Autodesk Fusion 360 part; units mm, degrees
sketch "Sketch1" plane through (0, 0, 0) normal (0, 0, 1) x (1, 0, 0)
  line L0 (110, 0) -> (80, 0)
  line L1 (80, 0) -> (80, 20)
  line L2 (80, 20) -> (40, 20)
  line L3 (40, 20) -> (40, 0)
  line L4 (0, 0) -> (40, 0)
  line L5 (80, 0) -> (110, 0)
  line L6 (110, 0) -> (110, 10)
  line L7 (110, 10) -> (90, 10)
  line L8 (90, 10) -> (90, 50)
  line L9 (90, 50) -> (20, 50)
  line L10 (0, 0) -> (0, 10)
  line L11 (0, 10) -> (20, 10)
  line L12 (20, 10) -> (20, 50)
  dimension "d1" = 110
  dimension "d2" = 30
  dimension "d3" = 20
  dimension "d4" = 40
  dimension "d5" = 10
  dimension "d6" = 20
  dimension "d7" = 70
  dimension "d8" = 10
  dimension "d9" = 20
extrude "Extrude1" add sketch "Sketch1" along normal blind 50
sketch "Sketch2" plane through (0, 0, 50) normal (0, 0, 1) x (1, 0, 0)
  line L0 (0, 0) -> (40, 0)
  line L1 (40, 0) -> (40, 20)
  line L2 (40, 20) -> (80, 20)
  line L3 (80, 20) -> (80, 0)
  line L4 (80, 0) -> (110, 0)
  line L5 (110, 0) -> (110, 10)
  line L6 (110, 10) -> (90, 10)
  line L7 (90, 10) -> (90, 50)
  line L8 (90, 50) -> (20, 50)
  line L9 (20, 50) -> (20, 10)
  line L10 (20, 10) -> (0, 10)
  line L11 (0, 10) -> (0, 0)
  line L12 (20, 50) -> (40, 50)
  line L13 (40, 50) -> (40, 40)
  line L14 (40, 40) -> (70, 40)
  line L15 (70, 40) -> (70, 50)
  line L16 (70, 50) -> (90, 50)
  dimension "d12" = 10
extrude "Extrude2" cut sketch "Sketch2" against normal blind 51 contours L8 L13 L14 L15
sketch "Sketch3" plane through (0, 50, 0) normal (0, 1, 0) x (-1, 0, 0)
  line L0 (-40, 50) -> (-40, 0)
  line L1 (-40, 0) -> (-20, 0)
  line L2 (-20, 0) -> (-20, 50)
  line L3 (-20, 50) -> (-40, 50)
  line L4 (-90, 0) -> (-90, 50)
  line L5 (-20, 40) -> (-90, 40)
  line L6 (-20, 10) -> (-90, 10)
  dimension "d15" = 10
  dimension "d16" = 10
extrude "Extrude3" cut sketch "Sketch3" against normal blind 20 contours L0 L2 L5 L6 | L0 L4 L5 L6
Input: part model. Units: mm. Frame: model coordinates. A direction names the side the tool comes from. Round coordinates to 2 decimals unless told otherwise and drop trailing zeros. Loops run counter-clockwise (first coordinate to the right, second up) from the corner with the lowest first, then second, coordinate; pieces in that order, holes last. Notation, with made-up numbers: (59.5, -8.75) -> (84.5, -8.75) arc R19 ccw to (84.5, 28.25) -> close; hole circle Ø5 at (87, -20.5). An arc over 180 degrees is marked (long way). Use one line per item in the form item = value. Start each with the question number.
Item 1: Section query D-D on y = 32. Return the cut outline in (x, z).
Item 2: Section query A-A on y = 46. Return the cut outline in (x, z), then the cut area to 3 significant figures.
Item 3: Section query B-B on x = 82. Return the cut outline in (y, z), then the cut area to 3 significant figures.
Item 4: Section query C-C on z = 14.5. Return the cut outline in (x, y), then the cut area to 3 significant figures.
Item 5: Set-up query: faces 5 (the face through (20, 25, 25)), 6 (the face through (40, 45, 45)), 7 (the face through (90, 25, 25)). Return all of +Z, -Z, +X, -X, +Y, -Y with unobstructed straight access to the full face (end or side cutting, diameter ignored); none if empty.
Item 6: Mould query, pull axis Z, two halves, no side actions, for faces 1 (the face through (40, 10, 25)), 2 (the face through (55, 38, 10)), 3 (the face through (55, 30, 25)), 4 (the face through (54, 25, 50)). Classes: pulls with the +Z half, pulls with the -Z half, needs draft (parallel to the pull), parting line crosses it, or undercut.
Item 7: Material intervals for L1, parallel to Z at x = 77, y = 30.5; L2, parallel to X at y = 8.5, z = 40; L3, parallel to X at y = 16.5, z = 25, sorted ascending. Write a range as from..to.
Item 8: Contact query for flat-ended pins moving along their axis: pin 1 Ø12 at (x, z) = (67.5, 16.5) entering from -Y; pin 2 Ø8 at (x, z) = (46.5, 19.5) entering from +Y; pin 3 Ø6 at (x, z) = (13.5, 21) entering from +Y. Output: stop coordinate, or through.
Ans:
q1.outline = (20, 0) -> (90, 0) -> (90, 10) -> (20, 10) -> close; (20, 40) -> (90, 40) -> (90, 50) -> (20, 50) -> close
q2.outline = (20, 0) -> (40, 0) -> (40, 10) -> (20, 10) -> close; (20, 40) -> (40, 40) -> (40, 50) -> (20, 50) -> close; (70, 0) -> (90, 0) -> (90, 10) -> (70, 10) -> close; (70, 40) -> (90, 40) -> (90, 50) -> (70, 50) -> close
q2.area = 800 mm^2
q3.outline = (0, 0) -> (50, 0) -> (50, 10) -> (30, 10) -> (30, 40) -> (50, 40) -> (50, 50) -> (0, 50) -> close
q3.area = 1,900 mm^2
q4.outline = (0, 0) -> (40, 0) -> (40, 20) -> (80, 20) -> (80, 0) -> (110, 0) -> (110, 10) -> (90, 10) -> (90, 30) -> (20, 30) -> (20, 10) -> (0, 10) -> close
q4.area = 1,700 mm^2
q5.face_5 = +Z, -Z, -X, +Y
q5.face_6 = +Z, -Z, +Y
q5.face_7 = +Z, -Z, +X, +Y
q6.face_1 = needs draft
q6.face_2 = undercut
q6.face_3 = undercut
q6.face_4 = pulls with the +Z half
q7.L1 = 0..10, 40..50
q7.L2 = 0..40, 80..110
q7.L3 = 20..40, 80..90
q8.pin_1 = 20
q8.pin_2 = 30
q8.pin_3 = 10
